from build123d import *

# Parameters (mm, degrees)
F1_DEPTH = 76.2
F4_D     = 12.7
F6_D     = 12.7


with BuildPart() as f1:
    # F0 (on Front) → F1 (new body)
    with BuildSketch(Plane.XZ):
        Polygon((0, 103.467127), (-50.8, 103.467127), (-50.8, -99.732873), (101.6, -99.732873), (101.6, -48.932873), (0, -48.932873), align=None)
    extrude(amount=F1_DEPTH)

    # F4 (through all)
    with Locations(Plane.YZ):
        with Locations((-38.1, 65.367127)):
            Hole(F4_D / 2)

    # F6 (through all)
    with Locations(Plane.XY.offset(-48.932873)):
        with Locations((63.5, -38.1)):
            Hole(F6_D / 2)


solid = f1.part
Could you check a few things on this model? Use its own coordinates, in mm. Coordinates: 2 decimals unless noted, no trailing zeros. Order: outer loops, then holes, each group sorted by start corner. A loop starts at its lowest first (then second) coordinate and runs counter-clockwise, first axis right, second up. Notation, with made-up numbers: (88, 31.25) -> (112, 31.25) arc R18 ccw to (112, 51.25) -> close; hole circle Ø7 at (88, 61.5). An arc over 180 degrees is marked (long way). One line per item, written item: value. Start each with the question number.
1) Imagine slicing it at A-A on y = -38.1. List the corners of the cut face in (x, z) for me.
2) Imagine slicing it at D-D on z = 86.5. List the corners of the cut face in (x, y) for me, plus the area to 3 significant figures.
3) I'm going to push flat-ended pins straight in: pin 1 (1 mm diameter, centred on y = -47, z = -4.5, fed in from +X); pin 2 (20.5 mm diameter, centred on x = 63.5, y = -38.1, fed in from +Z). Where does each tip first touch, or does it pass through?
4) If I drill on L1, parallel to Y at x = 63.5, z = -81; L2, parallel to Z at x = -20, y = -38.1; L3, parallel to X at y = -38, z = -78, over which ranges is the centre line in solid material (lowest first)? Write a range as [from, to].
5) Imagine slicing it at B-B on x = 63.5. List the corners of the cut face in (y, z) for me, plus the area to 3 significant figures.
6) We'd pull the mould along Z, two halves only. Please class faces 1 (the flat face through (0, -38, 26)), 2 (the flat face through (24, -38, -99.733)), 3 (the flat face through (52, -38, -48.933)), 4 (the cylindrical face through (-25.76, -33.42, 69.66)): +Z half, -Z half, draft (parallel to the pull), parting line (faces both ways), or undercut.
7) Imagine slicing it at C-C on y = -54. List the corners of the cut face in (x, z) for me.
Answer list:
1. outline: (-50.8, -99.73) -> (57.15, -99.73) -> (57.15, -48.93) -> (0, -48.93) -> (0, 59.02) -> (-50.8, 59.02) -> close; (-50.8, 71.72) -> (0, 71.72) -> (0, 103.47) -> (-50.8, 103.47) -> close; (69.85, -99.73) -> (101.6, -99.73) -> (101.6, -48.93) -> (69.85, -48.93) -> close
2. outline: (-50.8, -76.2) -> (0, -76.2) -> (0, 0) -> (-50.8, 0) -> close
2. area: 3,870 mm2
3. pin 1: stops at x = 0
3. pin 2: stops at z = -48.93
4. L1: y = [-76.2, -44.45], [-31.75, 0]
4. L2: z = [-99.73, 59.02], [71.72, 103.47]
4. L3: x = [-50.8, 57.15], [69.85, 101.6]
5. outline: (-76.2, -99.73) -> (-44.45, -99.73) -> (-44.45, -48.93) -> (-76.2, -48.93) -> close; (-31.75, -99.73) -> (0, -99.73) -> (0, -48.93) -> (-31.75, -48.93) -> close
5. area: 3,230 mm2
6. face 1: draft
6. face 2: -Z half
6. face 3: +Z half
6. face 4: undercut
7. outline: (-50.8, -99.73) -> (101.6, -99.73) -> (101.6, -48.93) -> (0, -48.93) -> (0, 103.47) -> (-50.8, 103.47) -> close
